Model file for the job. Use its own axes, mm. Face numbers are marked on the shaded views. A direction names the side the tool comes from. Give positions to 0.01 mm unless a question says otherwise; leave off trailing zeros. Order: outer loops, then holes, each group sorted by start corner. A loop starts at its lowest first (then second) coordinate and runs counter-clockwise, first axis right, second up. Notation, with made-up numbers: (-6, 79) -> (44, 79) arc R20 cw to (44, 95) -> close; hole circle Ø1 at (13, 85.5). An arc over 180 degrees is marked (long way). Use CSV: the item, a comma, the result in double quotes. Start each with the question number.
1. Wall check: line 1 (Z direction, x = -5, y = 4.5); line 2 (X direction, y = -8.5, z = -16); line 3 (Z direction, x = -0.5, y = 4.5). Give the ranges that are in metal, low to high. Write a range as from..to.
2. Cut at A-A on z = -14. List the corners of the cut face in (x, y), then the cut area to 3 significant figures.
3. Drop flat-ended pins along their axis: pin 1 (1 mm diameter, centred on x = -2.5, z = -15, fed in from -Y); pin 2 (10 mm diameter, centred on y = 0, z = -7, fed in from +X); pin 3 (5 mm diameter, centred on y = -4.61, z = -14, fed in from -X); pin 4 (4 mm diameter, centred on x = -0.08, y = -2.66, fed in from -Z). Give the stop position or say it passes through.
4. Cut at B-B on y = 9. List the corners of the cut face in (x, z), then the cut area to 3 significant figures.
5. 3-axis set-ups, long thin cutter, end or side, ignore diameter. For the marked faces 1 and 2: which of +Z, -Z, +X, -X, +Y, -Y reach the whole face in a straight line?
6. Cut at D-D on y = 6.25. List the corners of the cut face in (x, z).
7. Cut at C-C on x = -0.75. List the corners of the cut face in (y, z).
```python
from build123d import *

# Parameters (mm, degrees)
SKETCH_1_R          = 1.25
EXTRUDE_1_DEPTH     = 5
SKETCH_2_W          = 5
SKETCH_2_H          = 25
EXTRUDE_2_DEPTH     = 4
SKETCH_3_W          = 4
SKETCH_3_H          = 25
EXTRUDE_3_DEPTH     = 20
SKETCH_4_R          = 1.5
CUT_EXTRUDE_1_DEPTH = 20


with BuildPart() as part:
    # 草图1 → 凸台-拉伸1 (new body)
    with BuildSketch(Plane.XY):
        Polygon((-3.581151343, -8.027992706), (-3.581151343, -12.611885422), (2.918848657, -12.611885422), (2.918848657, -6.641886627), (2.918848657, 12.388114578), (-3.581151343, 12.388114578), align=None)
        with Locations((-0.081151343, 8.237522913)):
            Circle(SKETCH_1_R, mode=Mode.SUBTRACT)
        with Locations((-0.081151343, 2.787522913)):
            Circle(SKETCH_1_R, mode=Mode.SUBTRACT)
        with Locations((-0.081151343, -2.662477087)):
            Circle(SKETCH_1_R, mode=Mode.SUBTRACT)
        with Locations((-0.000846901, -8.111885422)):
            Circle(SKETCH_1_R, mode=Mode.SUBTRACT)
    extrude(amount=EXTRUDE_1_DEPTH)

    # 草图2 → 凸台-拉伸2 (add)
    with BuildSketch(Plane.ZY.offset(3.581151343)):
        with Locations((2.5, -0.111885422)):
            Rectangle(SKETCH_2_W, SKETCH_2_H)
    extrude(amount=EXTRUDE_2_DEPTH)

    # 草图3 → 凸台-拉伸3 (add)
    with BuildSketch(Plane(origin=(0, 0, 0), x_dir=(-1, 0, 0), z_dir=(0, 0, -1))):
        with Locations((5.581151343, -0.111885422)):
            Rectangle(SKETCH_3_W, SKETCH_3_H)
    extrude(amount=EXTRUDE_3_DEPTH)

    # 草图4 → 切除-拉伸1 (cut)
    with BuildSketch(Plane(origin=(-3.581151343, 0, 0), x_dir=(0, 0, -1), z_dir=(1, 0, 0))):
        with Locations(Location((6, 3.388114578, 0), (0, 0, 90))):
            Circle(SKETCH_4_R)
        with Locations(Location((14, 3.388114578, 0), (0, 0, 180))):
            Circle(SKETCH_4_R)
        with Locations(Location((14, -4.611885422, 0), (0, 0, 90))):
            Circle(SKETCH_4_R)
        with Locations(Location((6, -4.611885422, 0), (0, 0, 180))):
            Circle(SKETCH_4_R)
    extrude(amount=-CUT_EXTRUDE_1_DEPTH, mode=Mode.SUBTRACT)


solid = part.part
```
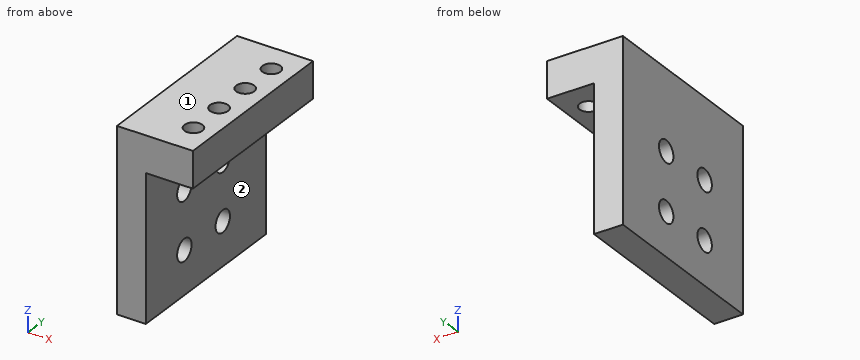
Verdict:
1,line 1,"-20..-15.01, -12.99..-7.01, -4.99..5"
1,line 2,"-7.58..-3.58"
1,line 3,"0..5"
2,outline,"(-7.58, -12.61) -> (-3.58, -12.61) -> (-3.58, -6.11) -> (-7.58, -6.11) -> close; (-7.58, -3.11) -> (-3.58, -3.11) -> (-3.58, 1.89) -> (-7.58, 1.89) -> close; (-7.58, 4.89) -> (-3.58, 4.89) -> (-3.58, 12.39) -> (-7.58, 12.39) -> close"
2,area,"76.0 mm^2"
3,pin 1,"through"
3,pin 2,"x = -3.58"
3,pin 3,"x = -7.58"
3,pin 4,"z = 0"
4,outline,"(-7.58, -20) -> (-3.58, -20) -> (-3.58, 0) -> (-1.07, 0) -> (-1.07, 5) -> (-7.58, 5) -> close; (0.91, 0) -> (2.92, 0) -> (2.92, 5) -> (0.91, 5) -> close"
4,area,"123 mm^2"
5,face 1,"+Z, +X, -X, +Y, -Y"
5,face 2,"-Z, +X, +Y, -Y"
6,outline,"(-7.58, -20) -> (-3.58, -20) -> (-3.58, 0) -> (2.92, 0) -> (2.92, 5) -> (-7.58, 5) -> close"
7,outline,"(-12.61, 0) -> (-9.11, 0) -> (-9.11, 5) -> (-12.61, 5) -> close; (-7.11, 0) -> (-3.72, 0) -> (-3.72, 5) -> (-7.11, 5) -> close; (-1.61, 0) -> (1.73, 0) -> (1.73, 5) -> (-1.61, 5) -> close; (3.84, 0) -> (7.18, 0) -> (7.18, 5) -> (3.84, 5) -> close; (9.29, 0) -> (12.39, 0) -> (12.39, 5) -> (9.29, 5) -> close"
